from build123d import *

# Parameters (mm, degrees)
SKETCH1_R           = 82.55
BOSS_EXTRUDE1_DEPTH = 3.175
SKETCH2_R           = 2.15
SKETCH2_W           = 40.6
SKETCH2_H           = 20.3
CUT_EXTRUDE1_DEPTH  = 3.175
SKETCH3_R           = 1.65
CUT_EXTRUDE2_DEPTH  = 3.175
CIRPATTERN1_COUNT   = 4
SKETCH4_R           = 46.35
SKETCH4_R_2         = 40
BOSS_EXTRUDE2_DEPTH = 4
SKETCH7_R           = 1.5875
SKETCH8_R           = 50.175
SKETCH8_R_2         = 47
BOSS_EXTRUDE3_DEPTH = 15


with BuildPart() as part:
    # Sketch1 → Boss-Extrude1 (new body)
    with BuildSketch(Plane(origin=(0, 0, 0), x_dir=(1, 0, 0), z_dir=(0, 1, 0))):
        with Locations(Location((0, 0, 0), (0, 0, 270))):
            Circle(SKETCH1_R)
    extrude(amount=BOSS_EXTRUDE1_DEPTH)

    # Sketch2 → Cut-Extrude1 (cut)
    with BuildSketch(Plane(origin=(0, 3.175, 0), x_dir=(1, 0, 0), z_dir=(0, 1, 0))):
        with Locations(Location((-24.15, 5, 0), (0, 0, 270))):
            Circle(SKETCH2_R)
        with Locations(Location((-24.15, -5, 0), (0, 0, 270))):
            Circle(SKETCH2_R)
        with Locations(Location((24.15, 5, 0), (0, 0, 270))):
            Circle(SKETCH2_R)
        with Locations(Location((24.15, -5, 0), (0, 0, 270))):
            Circle(SKETCH2_R)
        Rectangle(SKETCH2_W, SKETCH2_H)
    extrude(amount=-CUT_EXTRUDE1_DEPTH, mode=Mode.SUBTRACT)

    # Sketch3 → Cut-Extrude2 (cut)
    with BuildSketch(Plane(origin=(0, 3.175, 0), x_dir=(1, 0, 0), z_dir=(0, 1, 0))):
        with Locations(Location((-76.2, 0, 0), (0, 0, 270))):
            Circle(SKETCH3_R)
    cut_extrude2 = extrude(amount=-CUT_EXTRUDE2_DEPTH, mode=Mode.SUBTRACT)

    # CirPattern1: Cut-Extrude2 ×4 about axis
    cirpattern1_axis = Axis((0, 0, 0), (0, 1, 0))
    for i in range(1, CIRPATTERN1_COUNT):
        add(cut_extrude2.rotate(cirpattern1_axis, i * 360 / CIRPATTERN1_COUNT), mode=Mode.SUBTRACT)

    # Sketch4 → Boss-Extrude2 (add)
    with BuildSketch(Plane(origin=(0, 3.175, 0), x_dir=(1, 0, 0), z_dir=(0, 1, 0))):
        with Locations(Location((-9.65, 0, 0), (0, 0, 270))):
            Circle(SKETCH4_R)
        with Locations(Location((-9.65, 0, 0), (0, 0, 270))):
            Circle(SKETCH4_R_2, mode=Mode.SUBTRACT)
    extrude(amount=BOSS_EXTRUDE2_DEPTH)

    # Sketch7 → Cut-Revolve1 (revolve, cut)
    with BuildSketch(Plane.XY, mode=Mode.PRIVATE) as cut_revolve1_sk:
        with Locations((-52.825, 7.675)):
            Circle(SKETCH7_R)
    revolve(cut_revolve1_sk.sketch.rotate(Axis((-9.65, 3.175, 0), (0, 1, 0)), 270), axis=Axis((-9.65, 3.175, 0), (0, 1, 0)), mode=Mode.SUBTRACT)

    # Sketch8 → Boss-Extrude3 (add)
    with BuildSketch(Plane(origin=(0, 3.175, 0), x_dir=(1, 0, 0), z_dir=(0, 1, 0))):
        with Locations(Location((-9.65, 0, 0), (0, 0, 270))):
            Circle(SKETCH8_R)
        with Locations(Location((-9.65, 0, 0), (0, 0, 270))):
            Circle(SKETCH8_R_2, mode=Mode.SUBTRACT)
    extrude(amount=BOSS_EXTRUDE3_DEPTH)


solid = part.part
The listing builds one solid part. Answer for the finished solid, in the listing's coordinates (mm). A direction names the side the tool comes from. Give positions to 0.01 mm unless a question says otherwise; leave off trailing zeros. Order: outer loops, then holes, each group sorted by start corner. A loop starts at its lowest first (then second) coordinate and runs counter-clockwise, first axis right, second up. Notation, with made-up numbers: (66, 1.5) - (111, 1.5) arc R11 ccw to (111, 13.5) - close; hole circle Ø3 at (-22, 43). An arc over 180 degrees is marked (long way). Use one line per item in the form item = value.
1) For faces 1 (the cylindrical face through (-22, 2, -5)), 2 (the cylindrical face through (-48.7, 5.15, -8.67)), determine the directions among +Z, -Z, +X, -X, +Y, -Y from which every point of the face is accessible in a straight line to the end or side of a thin tool.
Verdict:
face_1 = +Y, -Y
face_2 = +Y
2) Find section D-D on z = 58. Determine the outline of the cut face in (x, y) (3 decimals), and give its area (3 significant figures).
Verdict:
outline = (-58.741, 0) - (58.741, 0) - (58.741, 3.175) - (-58.741, 3.175) - close
area = 373 mm^2
3) Each of these flat-tipped pins is pushed along its axis until it touches: pin 1 (2.5 mm diameter, centred on x = 24.15, z = 5, fed in from -Y); pin 2 (1.5 mm diameter, centred on y = 6.5, z = -26, fed in from +X); pin 3 (2.5 mm diameter, centred on x = 5.5, y = 1, fed in from +Z); pin 4 (6 mm diameter, centred on y = 5.5, z = -62.5, fed in from -X). Where does it stop, or does it pass through?
Verdict:
pin_1 = through
pin_2 = 33.71
pin_3 = 82.44
pin_4 = -56.05
4) Find section B-B on y = 9.25. Determine the outline of the cut face in (x, z) (3 decimals), and give its area (3 significant figures).
Verdict:
outline = circle Ø100.35 at (-9.65, 0); hole circle Ø94 at (-9.65, 0)
area = 969 mm^2
5) Find section C-C on x = 24.15. Give the number of separate pieces and of enclosed holes in the cut face, and give its area (3 significant figures).
Verdict:
separate_pieces = 3
enclosed_holes = 0
area = 682 mm^2
6) The mould has two halves that part along X. Classify faces 3 (the cylindrical face through (-54.164, 10.57, 23.153)), 4 (the cylindrical face through (22.842, 1.61, 3.294)), 5 (the flat face through (-24, 18.175, -45)), 6 (the flat face through (28, 7.175, -16)): released by +X, released by -X, zero draft, split by the parting line, or undercut.
Verdict:
face_3 = split by the parting line
face_4 = undercut
face_5 = zero draft
face_6 = undercut
7) Consider probe 1 along Z at (x, y) = (1.5, 1.25); probe 2 along X at (y, z) = (1.85, 5); probe 3 along X at (y, z) = (5, -3.5). Determine where each line is inside the solid, lowest interval first. Write a range as [from, to].
Verdict:
probe_1 = [-82.54, -76.89], [-75.51, -10.15], [10.15, 75.51], [76.89, 82.54]
probe_2 = [-82.4, -26.3], [-22, -20.3], [20.3, 22], [26.3, 82.4]
probe_3 = [-59.7, -56.52], [-55.87, -49.5], [30.2, 36.57], [37.22, 40.4]
